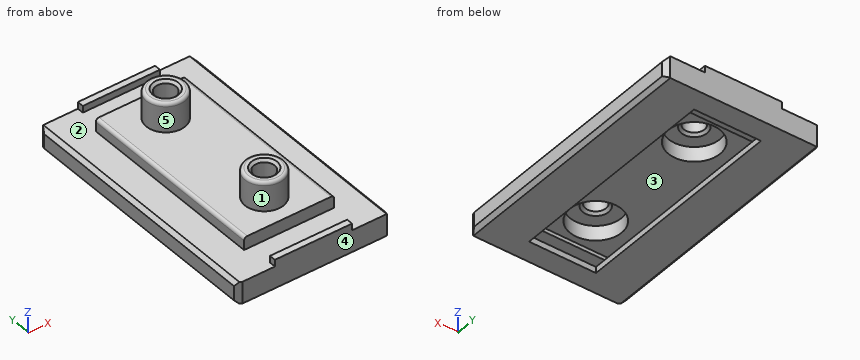
```python
from build123d import *
from OCP.BRepFilletAPI import BRepFilletAPI_MakeChamfer

# Parameters (mm, degrees)
ESQUISSE1_W                                        = 23.9
ESQUISSE1_H                                        = 40
BOSS_EXTRU_1_DEPTH                                 = 3.4
ENL_V_MAT_EXTRU_1_DEPTH                            = 30
ESQUISSE3_W                                        = 14
ESQUISSE3_H                                        = 30.1
BOSS_EXTRU_2_DEPTH                                 = 1.95
ESQUISSE4_W                                        = 10.4
ESQUISSE4_H                                        = 30
ENL_V_MAT_EXTRU_2_DEPTH                            = 1.55
ENL_V_MAT_EXTRU_3_REACH                            = 25.71
ESQUISSE6_W                                        = 10.4
ESQUISSE6_H                                        = 1.75
ENL_V_MAT_EXTRU_4_REACH                            = 25.71
ESQUISSE8_W                                        = 10.4
ESQUISSE8_H                                        = 1.75
ESQUISSE9_W                                        = 0.6
ESQUISSE9_H                                        = 30
ENL_V_MAT_EXTRU_5_DEPTH                            = 1.8
ESQUISSE10_W                                       = 0.6
ESQUISSE10_H                                       = 30
ENL_V_MAT_EXTRU_6_DEPTH                            = 1.8
ESQUISSE11_W                                       = 12
ESQUISSE11_H                                       = 1
BOSS_EXTRU_3_DEPTH                                 = 1.05
ESQUISSE12_W                                       = 12
ESQUISSE12_H                                       = 1
BOSS_EXTRU_4_DEPTH                                 = 1.05
ESQUISSE13_W                                       = 3
ESQUISSE13_H                                       = 4.5
ESQUISSE14_W                                       = 3
ESQUISSE14_H                                       = 4.5
CHAMBRAGE_POUR_VIS_T_TE_HEXAGONALE_M31_D           = 3.2
CHAMBRAGE_POUR_VIS_T_TE_HEXAGONALE_M31_CBORE_D     = 8
CHAMBRAGE_POUR_VIS_T_TE_HEXAGONALE_M31_CBORE_DEPTH = 2.3
CHANFREIN1_SIZE                                    = 0.913344887
CHANFREIN1_SIZE2                                   = 0.527
CHANFREIN2_SIZE                                    = 0.527
CHANFREIN2_SIZE2                                   = 0.913344887
CHANFREIN3_SIZE                                    = 0.577
CHANFREIN4_SIZE                                    = 0.4
CONG_1_R                                           = 0.5


with BuildPart() as part:
    # Esquisse1 → Boss.-Extru.1 (new body)
    with BuildSketch(Plane.XY.offset(7.55)):
        Rectangle(ESQUISSE1_W, ESQUISSE1_H)
    extrude(amount=-BOSS_EXTRU_1_DEPTH)

    # Esquisse2 → Enlèv. mat.-Extru.1 (cut)
    with BuildSketch(Plane(origin=(0, 15, 0), x_dir=(1, 0, 0), z_dir=(0, 1, 0))):
        with BuildLine():
            Line((6.995, -7.4), (6.995, -7.55))
            Line((6.995, -7.55), (7, -7.55))
            Line((7, -7.55), (7, -7.310697145))
            ThreePointArc((7, -7.310697145), (6.996250978, -7.35527864), (6.995, -7.4))
        make_face()
    extrude(amount=-ENL_V_MAT_EXTRU_1_DEPTH, mode=Mode.SUBTRACT)

    # Esquisse3 → Boss.-Extru.2 (add)
    with BuildSketch(Plane.XY.offset(7.55)):
        with Locations((-0.005, 0)):
            Rectangle(ESQUISSE3_W, ESQUISSE3_H)
    extrude(amount=BOSS_EXTRU_2_DEPTH)

    # Esquisse4 → Enlèv. mat.-Extru.2 (cut)
    with BuildSketch(Plane(origin=(0, 0, 4.15), x_dir=(-1, 0, 0), z_dir=(0, 0, -1))):
        Rectangle(ESQUISSE4_W, ESQUISSE4_H)
    extrude(amount=-ENL_V_MAT_EXTRU_2_DEPTH, mode=Mode.SUBTRACT)

    # Esquisse6 → Enlèv. mat.-Extru.3 (cut, up to next)
    with BuildSketch(Plane.XY.offset(5.1), mode=Mode.PRIVATE) as enl_v_mat_extru_3_sk1:
        with Locations((0, -15.875)):
            Rectangle(ESQUISSE6_W, ESQUISSE6_H)
    enl_v_mat_extru_3_tool1 = extrude(enl_v_mat_extru_3_sk1.sketch, amount=-ENL_V_MAT_EXTRU_3_REACH, mode=Mode.PRIVATE) & part.part
    add(enl_v_mat_extru_3_tool1.solids().sort_by_distance((0, -15.875, 5.1))[0], mode=Mode.SUBTRACT)

    # Esquisse8 → Enlèv. mat.-Extru.4 (cut, up to next)
    with BuildSketch(Plane.XY.offset(5.1), mode=Mode.PRIVATE) as enl_v_mat_extru_4_sk1:
        with Locations((0, 15.875)):
            Rectangle(ESQUISSE8_W, ESQUISSE8_H)
    enl_v_mat_extru_4_tool1 = extrude(enl_v_mat_extru_4_sk1.sketch, amount=-ENL_V_MAT_EXTRU_4_REACH, mode=Mode.PRIVATE) & part.part
    add(enl_v_mat_extru_4_tool1.solids().sort_by_distance((0, 15.875, 5.1))[0], mode=Mode.SUBTRACT)

    # Esquisse9 → Enlèv. mat.-Extru.5 (cut)
    with BuildSketch(Plane.ZY.offset(-5.2)):
        with Locations((5.4, 0)):
            Rectangle(ESQUISSE9_W, ESQUISSE9_H)
    extrude(amount=-ENL_V_MAT_EXTRU_5_DEPTH, mode=Mode.SUBTRACT)

    # Esquisse10 → Enlèv. mat.-Extru.6 (cut)
    with BuildSketch(Plane(origin=(-5.2, 0, 0), x_dir=(0, 0, -1), z_dir=(1, 0, 0))):
        with Locations((-5.4, 0)):
            Rectangle(ESQUISSE10_W, ESQUISSE10_H)
    extrude(amount=-ENL_V_MAT_EXTRU_6_DEPTH, mode=Mode.SUBTRACT)

    # Esquisse11 → Boss.-Extru.3 (add)
    with BuildSketch(Plane.XY.offset(7.55)):
        with Locations((0, -19.5)):
            Rectangle(ESQUISSE11_W, ESQUISSE11_H)
    extrude(amount=BOSS_EXTRU_3_DEPTH)

    # Esquisse12 → Boss.-Extru.4 (add)
    with BuildSketch(Plane.XY.offset(7.55)):
        with Locations((0, 19.5)):
            Rectangle(ESQUISSE12_W, ESQUISSE12_H)
    extrude(amount=BOSS_EXTRU_4_DEPTH)

    # Esquisse13 → Révolution1 (revolve)
    with BuildSketch(Plane.XZ.offset(-10), mode=Mode.PRIVATE) as r_volution1_sk:
        with Locations((1.5, 11.75)):
            Rectangle(ESQUISSE13_W, ESQUISSE13_H)
    revolve(r_volution1_sk.sketch.rotate(Axis((0, 10, 14), (0, 0, -1)), 180), axis=Axis((0, 10, 14), (0, 0, -1)))

    # Esquisse14 → Révolution2 (revolve)
    with BuildSketch(Plane.XZ.offset(10), mode=Mode.PRIVATE) as r_volution2_sk:
        with Locations((1.5, 11.75)):
            Rectangle(ESQUISSE14_W, ESQUISSE14_H)
    revolve(r_volution2_sk.sketch.rotate(Axis((0, -10, 14), (0, 0, -1)), 180), axis=Axis((0, -10, 14), (0, 0, -1)))

    # Chambrage pour vis à tête hexagonale M31 (through all)
    with Locations(Plane(origin=(0, 0, 5.7), x_dir=(-1, 0, 0), z_dir=(0, 0, -1))):
        with Locations((0, -10), (0, 10)):
            CounterBoreHole(CHAMBRAGE_POUR_VIS_T_TE_HEXAGONALE_M31_D / 2, CHAMBRAGE_POUR_VIS_T_TE_HEXAGONALE_M31_CBORE_D / 2, CHAMBRAGE_POUR_VIS_T_TE_HEXAGONALE_M31_CBORE_DEPTH)

    # Chanfrein1
    chanfrein1_edges = [part.edges().sort_by_distance(p)[0] for p in [
        (11.95, 20, 5.85),
    ]]
    chanfrein1_side = [part.faces().sort_by_distance(p)[0] for p in [
        (11.95, 0, 5.85),
    ]]
    chamfer(chanfrein1_edges, length=CHANFREIN1_SIZE, length2=CHANFREIN1_SIZE2, reference=chanfrein1_side[0])

    # Chanfrein2: one chamfer whose edges measure the first distance from different faces: ONE call of the kernel's chamfer builder (chamfer() names one face for all edges)
    chanfrein2_edges_1 = [part.edges().sort_by_distance(p)[0] for p in [
        (11.95, -20, 5.85),
    ]]
    chanfrein2_side_1 = [part.faces().sort_by_distance(p)[0] for p in [
        (0, -20, 6.148689538),
    ]]
    chanfrein2_edges_2 = [part.edges().sort_by_distance(p)[0] for p in [
        (-11.95, -20, 5.85),
    ]]
    chanfrein2_side_2 = [part.faces().sort_by_distance(p)[0] for p in [
        (-11.95, 0, 5.85),
    ]]
    chanfrein2_edges_3 = [part.edges().sort_by_distance(p)[0] for p in [
        (-11.95, 20, 5.85),
    ]]
    chanfrein2_side_3 = [part.faces().sort_by_distance(p)[0] for p in [
        (-0.227438689, 20, 6.154502532),
    ]]
    chanfrein2 = BRepFilletAPI_MakeChamfer(part.part.solid().wrapped)
    for e in chanfrein2_edges_1:
        chanfrein2.Add(CHANFREIN2_SIZE, CHANFREIN2_SIZE2, e.wrapped, chanfrein2_side_1[0].wrapped)  # the first distance lies on this face
    for e in chanfrein2_edges_2:
        chanfrein2.Add(CHANFREIN2_SIZE, CHANFREIN2_SIZE2, e.wrapped, chanfrein2_side_2[0].wrapped)  # the first distance lies on this face
    for e in chanfrein2_edges_3:
        chanfrein2.Add(CHANFREIN2_SIZE, CHANFREIN2_SIZE2, e.wrapped, chanfrein2_side_3[0].wrapped)  # the first distance lies on this face
    add(Compound.cast(chanfrein2.Shape()), mode=Mode.REPLACE)

    # Chanfrein3
    chanfrein3_edges = [part.edges().sort_by_distance(p)[0] for p in [
        (-11.95, -0.193172444, 4.15),
        (-11.95, -0.193172444, 7.55),
        (11.95, 0, 4.15),
        (11.95, 0, 7.55),
    ]]
    chamfer(chanfrein3_edges, length=CHANFREIN3_SIZE)

    # Chanfrein4
    chanfrein4_edges = [part.edges().sort_by_distance(p)[0] for p in [
        (-1.6, 10, 14),
        (-1.6, 10, 8),
        (-1.6, -10, 14),
        (-1.6, -10, 8),
    ]]
    chamfer(chanfrein4_edges, length=CHANFREIN4_SIZE)

    # Congé1
    cong_1_edges = [part.edges().sort_by_distance(p)[0] for p in [
        (3, 10, 14),
        (3, -10, 14),
        (-7.005, 0, 9.5),
        (6.995, 0, 9.5),
    ]]
    fillet(cong_1_edges, radius=CONG_1_R)


solid = part.part
```
The listing builds one solid part. Answer for the finished solid, in the listing's coordinates (mm). Face numbers are marked on the shaded views. A direction names the side the tool comes from. Coordinates: 2 decimals unless noted, no trailing zeros. Write each loop counter-clockwise with the first axis right and the second up, starting at its lowest first coordinate (ties: lowest second). Pieces come first, ordered by that corner, then holes.
Q1. Which of the six approach directions +Z, -Z, +X, -X, +Y, -Y give full straight-line access (tool end or side, diameter ignored) to the marked faces 4 and 5?
Returned:
face 4: +Z, -Z, +X, -X, -Y
face 5: +Z
Q2. Given P1, Ø5, axis at x = 8.5, z = 12, coming from the +Y side; P2, Ø0.8, axis at y = 19.5, z = 8, coming from the +X side; P3, Ø1, axis at x = 8, y = 1.5, coming from the +Z side; P4, Ø1.6, axis at y = -7.5, z = 8, coming from the -X side, each flat-ended and moving along its own axis, determine where each tip first touches the part or whether it passes through.
Returned:
P1: passes through
P2: stops at x = 6
P3: stops at z = 7.55
P4: stops at x = -11.72
Q3. Section A-A, the plane x = -10.25 is taken. Write down the section's boundary in (y, z), then the cut area to 3 significant figures.
Returned:
outline: (-20, 4.15) - (20, 4.15) - (20, 7.55) - (-20, 7.55) - close
area: 136 mm2
Q4. Find the intervals of material crossed by line 1 along Y through (x, z) = (0, 10.15); line 2 along Y through (x, z) = (0, 6.65); line 3 along Z through (x, y) = (-6.5, 13.5), in increasing order.
Returned:
line 1: y = -13 to -11.6, -8.4 to -7, 7 to 8.4, 11.6 to 13
line 2: y = -20 to -14, -6 to 6, 14 to 20
line 3: z = 4.15 to 5.1, 5.7 to 9.5
Q5. Section B-B, the plane x = 0 is taken. Give the number of separate pieces and of enclosed holes in the cut face, then the cut area to 3 significant figures.
Returned:
separate pieces: 3
enclosed holes: 0
area: 125 mm2
Q6. The mould has two halves that part along X. Classify the marked faces 1, 2 and 3: released by +X, released by -X, zero draft, split by the parting line, or undercut.
Returned:
face 1: split by the parting line
face 2: zero draft
face 3: undercut
